Here's how the part is built. I have some questions about the finished solid (model axes, mm). A direction names the side the tool comes from. Give positions to 0.01 mm unless a question says otherwise; leave off trailing zeros. Loops run counter-clockwise (first coordinate to the right, second up) from the corner with the lowest first, then second, coordinate; pieces in that order, holes last. Notation, with made-up numbers: M 85.5,-30.5 L 120.5,-30.5 A21 cw 120.5,2.5 Z; hole C 2,68 d9. An arc over 180 degrees is marked long. Answer as CSV lines item,"result". Start each with the question number.
Item 1: I want a section at B-B on y = -24.75. List the corners of the cut face in (x, z) for me (3 decimals).
Item 2: I want a section at A-A on z = 4.9. List the corners of the cut face in (x, y) for me (3 decimals).
Item 3: If we mould it in two halves opening along Z, with no side actions, what happens to faces 6 (the flat face through (70, 30.6, 10)), 7 (the cylindrical face through (69.985, -22.627, 4.993)), 8 (the cylindrical face through (60.875, 13.371, 12.666))? For each: released by +Z, released by -Z, zero draft, split by the parting line, or undercut.
Item 4: If I drill on line 1 along Z through (x, y) = (70.55, 27.5) (3 decimals); line 2 along X through (y, z) = (10, 4); line 3 along Y through (x, z) = (75, 15.75), over which ranges is the centre line in solid material (lowest first)? Write a range as from..to.
Item 5: Will these pins go through, and if not, where does the flat tip stop? P1, Ø4, axis at x = 74, z = 7.5, coming from the +Y side; P2, Ø3, axis at y = -12.5, z = 14, coming from the -X side; P3, Ø5.5, axis at y = -25.5, z = 7.5, coming from the -X side; P4, Ø4, axis at y = -24.75, z = 4.9, coming from the -X side.
Item 6: I want a section at D-D on x = 72. List the corners of the cut face in (y, z) for me.
Item 7: For faces 1 (the cylindrical face through (69.985, 26.358, 16.692)), 2 (the flat face through (68.9, -24, 10)), 3 (the flat face through (85, 23.5, 10)), 4 (the flat face through (85, -20.75, 10)), 5 (the flat face through (66, 23.5, 10)), which set-ups out of +Z, -Z, +X, -X, +Y, -Y let a thin tool reach every point of the face, with its end or its side?
Item 8: I want a section at C-C on y = 12.5. List the corners of the cut face in (x, z) for me.
from build123d import *

# Parameters (mm, degrees)
SCHIZZO1_W                   = 40.3
SCHIZZO1_H                   = 44.25
ESTRUSIONE_ESTRUSIONE1_DEPTH = 19.8
SCHIZZO2_W                   = 19.8
SCHIZZO2_H                   = 44.25
SCHIZZO2_R                   = 2.9
TAGLIO_ESTRUSIONE1_DEPTH     = 3.6
SCHIZZO3_W                   = 2.2
SCHIZZO3_H                   = 19.8
ESTRUSIONE_ESTRUSIONE2_DEPTH = 7.1
SCHIZZO4_W                   = 2.2
SCHIZZO4_H                   = 19.8
ESTRUSIONE_ESTRUSIONE3_DEPTH = 7.1
SCHIZZO5_R                   = 2.125
TAGLIO_ESTRUSIONE2_DEPTH     = 7.1


with BuildPart() as part:
    # Schizzo1 → Estrusione-Estrusione1 (new body)
    with BuildSketch(Plane(origin=(0, 0, 0), x_dir=(-1, 0, 0), z_dir=(0, 0, 1))):
        with Locations((-79.25, -1.375)):
            Rectangle(SCHIZZO1_W, SCHIZZO1_H)
    extrude(amount=ESTRUSIONE_ESTRUSIONE1_DEPTH)

    # Schizzo2 → Taglio-Estrusione1 (cut)
    with BuildSketch(Plane.ZY.offset(-59.1)):
        with Locations((9.9, 1.375)):
            Rectangle(SCHIZZO2_W, SCHIZZO2_H)
        with Locations((9.9, 12.5)):
            Circle(SCHIZZO2_R, mode=Mode.SUBTRACT)
    extrude(amount=-TAGLIO_ESTRUSIONE1_DEPTH, mode=Mode.SUBTRACT)

    # Schizzo3 → Estrusione-Estrusione2 (add)
    with BuildSketch(Plane(origin=(0, 23.5, 0), x_dir=(1, 0, 0), z_dir=(0, 1, 0))):
        with Locations((70, -9.9)):
            Rectangle(SCHIZZO3_W, SCHIZZO3_H)
    extrude(amount=ESTRUSIONE_ESTRUSIONE2_DEPTH)

    # Schizzo4 → Estrusione-Estrusione3 (add)
    with BuildSketch(Plane.XZ.offset(20.75)):
        with Locations((70, 9.9)):
            Rectangle(SCHIZZO4_W, SCHIZZO4_H)
    extrude(amount=ESTRUSIONE_ESTRUSIONE3_DEPTH)

    # Schizzo5 → Taglio-Estrusione2 (cut)
    with BuildSketch(Plane.ZY.offset(-68.9)):
        with Locations(Location((14.9, 27.5, 0), (0, 0, 270))):
            Circle(SCHIZZO5_R)
        with Locations(Location((4.9, 27.5, 0), (0, 0, 270))):
            Circle(SCHIZZO5_R)
        with Locations(Location((14.9, -24.75, 0), (0, 0, 270))):
            Circle(SCHIZZO5_R)
        with Locations(Location((4.9, -24.75, 0), (0, 0, 270))):
            Circle(SCHIZZO5_R)
    extrude(amount=-TAGLIO_ESTRUSIONE2_DEPTH, mode=Mode.SUBTRACT)


solid = part.part
Result:
1,outline,"M 68.9,0 L 71.1,0 L 71.1,2.775 L 68.9,2.775 Z; M 68.9,7.025 L 71.1,7.025 L 71.1,12.775 L 68.9,12.775 Z; M 68.9,17.025 L 71.1,17.025 L 71.1,19.8 L 68.9,19.8 Z"
2,outline,"M 62.7,-20.75 L 68.9,-20.75 L 68.9,-22.625 L 71.1,-22.625 L 71.1,-20.75 L 99.4,-20.75 L 99.4,23.5 L 71.1,23.5 L 71.1,25.375 L 68.9,25.375 L 68.9,23.5 L 62.7,23.5 Z; M 68.9,-27.85 L 71.1,-27.85 L 71.1,-26.875 L 68.9,-26.875 Z; M 68.9,29.625 L 71.1,29.625 L 71.1,30.6 L 68.9,30.6 Z"
3,face 6,"zero draft"
3,face 7,"undercut"
3,face 8,"split by the parting line"
4,line 1,"0..2.775, 7.025..12.775, 17.025..19.8"
4,line 2,"62.7..99.4"
4,line 3,"-20.75..23.5"
5,P1,"y = 23.5"
5,P2,"x = 62.7"
5,P3,"x = 68.9"
5,P4,"through"
6,outline,"M -20.75,0 L 23.5,0 L 23.5,19.8 L -20.75,19.8 Z"
7,face 1,"+X, -X"
7,face 2,"+Z, -Z, -X, -Y"
7,face 3,"+Z, -Z, +X, +Y"
7,face 4,"+Z, -Z, +X, -Y"
7,face 5,"+Z, -Z, -X, +Y"
8,outline,"M 59.1,7 L 62.7,7 L 62.7,0 L 99.4,0 L 99.4,19.8 L 62.7,19.8 L 62.7,12.8 L 59.1,12.8 Z"
